The listing builds one solid part. Answer for the finished solid, in the listing's coordinates (mm). Coordinates: 2 decimals unless noted, no trailing zeros. Write each loop counter-clockwise with the first axis right and the second up, starting at its lowest first coordinate (ties: lowest second). Pieces come first, ordered by that corner, then holes.
from build123d import *

# Parameters (mm, degrees)
SKETCH_W      = 65
SKETCH_H      = 65
PAD_DEPTH     = 5
SKETCH001_R   = 1.75
SKETCH001_R_2 = 26
POCKET_DEPTH  = 5
FILLET_R      = 5


with BuildPart() as part:
    # Sketch → Pad (new body)
    with BuildSketch(Plane.XY):
        Rectangle(SKETCH_W, SKETCH_H)
    extrude(amount=PAD_DEPTH)

    # Sketch001 → Pocket (cut)
    with BuildSketch(Plane.XY):
        with Locations((-22.5, 22.754121)):
            Circle(SKETCH001_R)
        with Locations((22.5, 22.754121)):
            Circle(SKETCH001_R)
        with Locations((-22.5, -22.754121)):
            Circle(SKETCH001_R)
        with Locations((22.5, -22.754121)):
            Circle(SKETCH001_R)
        Circle(SKETCH001_R_2)
    extrude(amount=POCKET_DEPTH, mode=Mode.SUBTRACT)

    # Fillet
    fillet_edges = [part.edges().sort_by_distance(p)[0] for p in [
        (-32.5, -32.5, 2.5),
        (32.5, -32.5, 2.5),
        (32.5, 32.5, 2.5),
        (-32.5, 32.5, 2.5),
    ]]
    fillet(fillet_edges, radius=FILLET_R)


solid = part.part
Q1. The part is cut by section D-D, the plane y = 23.5. Write down the section's boundary in (x, z).
Answers below:
outline: (-32.5, 0) - (-24.08, 0) - (-24.08, 5) - (-32.5, 5) - close; (-20.92, 0) - (-11.12, 0) - (-11.12, 5) - (-20.92, 5) - close; (11.12, 0) - (20.92, 0) - (20.92, 5) - (11.12, 5) - close; (24.08, 0) - (32.5, 0) - (32.5, 5) - (24.08, 5) - close
Q2. Determine the mould class of faces 1 (the face through (0, 32.5, 2)), 2 (the face through (20.75, 22.83, 2.46)), 3 (the face through (-22, 15, 5)) for opening direction Y: released by +Y, released by -Y, zero draft, split by the parting line, or undercut.
Answers below:
face 1: released by +Y
face 2: undercut
face 3: zero draft
Q3. Find the intervals of material crossed by probe 1 along Y at (x, z) = (0, 2.1); probe 2 along Y at (x, z) = (21.5, 0.5); probe 3 along Y at (x, z) = (22.5, 1.1), in increasing order.
Answers below:
probe 1: y = -32.5 to -26, 26 to 32.5
probe 2: y = -32.5 to -24.19, -21.32 to -14.62, 14.62 to 21.32, 24.19 to 32.5
probe 3: y = -32.5 to -24.5, -21 to -13.03, 13.03 to 21, 24.5 to 32.5
Q4. Given pin 1 (3 mm diameter, centred on x = 22.5, y = 22.75, fed in from +Z), flat-ended and moving along its own axis, determine where the tip first touches the part or whether it passes through.
Answers below:
pin 1: passes through
Q5. The part is cut by section A-A, the plane x = 0. Write down the section's boundary in (y, z), then the cut area to 3 significant figures.
Answers below:
outline: (-32.5, 0) - (-26, 0) - (-26, 5) - (-32.5, 5) - close; (26, 0) - (32.5, 0) - (32.5, 5) - (26, 5) - close
area: 65.0 mm2
Q6. The part is cut by section C-C, the plane z = 2.55. Write down the section's boundary in (x, y).
Answers below:
outline: (-32.5, -27.5) arc R5 ccw to (-27.5, -32.5) - (27.5, -32.5) arc R5 ccw to (32.5, -27.5) - (32.5, 27.5) arc R5 ccw to (27.5, 32.5) - (-27.5, 32.5) arc R5 ccw to (-32.5, 27.5) - close; hole circle Ø52 at (0, 0); hole circle Ø3.5 at (-22.5, -22.75); hole circle Ø3.5 at (-22.5, 22.75); hole circle Ø3.5 at (22.5, -22.75); hole circle Ø3.5 at (22.5, 22.75)
